Geometry check sheet. Reference: the model listing, model coordinates, mm. Face numbers are marked on the shaded views. Round coordinates to 2 decimals unless told otherwise and drop trailing zeros. Order: outer loops, then holes, each group sorted by start corner. A loop starts at its lowest first (then second) coordinate and runs counter-clockwise, first axis right, second up. Notation, with made-up numbers: (11.25, 46) - (43.25, 46) arc R8 ccw to (43.25, 52) - close; hole circle Ø10 at (40, 48). An arc over 180 degrees is marked (long way). Use a Markdown table: item, result. Add a question column.
(1) Section check D-D on x = 28.5. Record the boundary of the cut face in (y, z).
(2) Section check B-B on y = -22. Record the boundary of the cut face in (x, z), then the cut area to 3 significant figures.
(3) Gauge pin test, flat ends, axial feed: P1, Ø2, axis at y = 51.5, z = 2.5, coming from the -X side; P2, Ø1.5, axis at x = -49.5, z = 5, coming from the +Y side. Record the tip position at first contact, or that the pin passes through.
(4) Section check A-A on x = 0. Record the boundary of the cut face in (y, z).
(5) Mould release check, pull along X, two halves, no side actions. Record for the marked faces 1 and 2: released by +X, released by -X, zero draft, split by the parting line, or undercut.
(6) Thickness scan on line 1 along Z through (x, y) = (-29, 20); line 2 along Y through (x, z) = (7, 4.55); line 3 along Y through (x, z) = (15, 4.35). Record the ranges inside material, lowest first. Write a range as [from, to].
(7) Section check C-C on z = 1.65. Record the boundary of the cut face in (x, y).
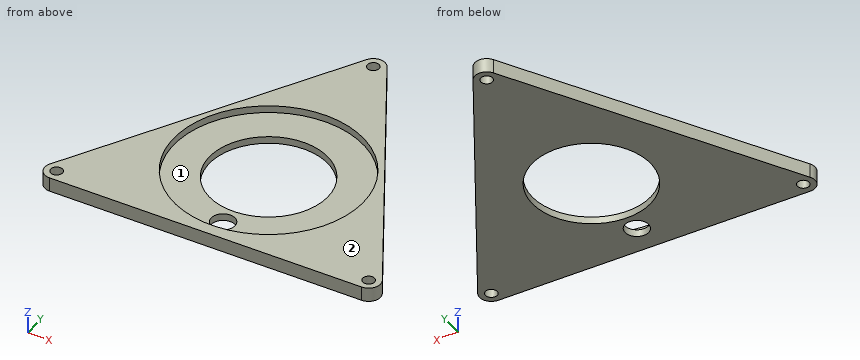
```python
from build123d import *

# Parameters (mm, degrees)
F0_R     = 2.5
F1_DEPTH = 6
F2_R     = 40
F3_DEPTH = 3
F4_R     = 25
F5_DEPTH = 25
F6_R     = 5
F7_DEPTH = 25


with BuildPart() as f1:
    # F0 (on Top) → F1 (new body)
    with BuildSketch(Plane.XY):
        with BuildLine():
            ThreePointArc((4.330127, 72.403811), (0, 74.903811), (-4.330127, 72.403811))
            Line((-4.330127, 72.403811), (-70.669873, -42.5))
            ThreePointArc((-70.669873, -42.5), (-70.669873, -47.5), (-66.339746, -50))
            Line((-66.339746, -50), (66.339746, -50))
            ThreePointArc((66.339746, -50), (70.669873, -47.5), (70.669873, -42.5))
            Line((70.669873, -42.5), (4.330127, 72.403811))
        make_face()
        with Locations((-66.339746, -45)):
            Circle(F0_R, mode=Mode.SUBTRACT)
        with Locations((66.339746, -45)):
            Circle(F0_R, mode=Mode.SUBTRACT)
        with Locations((0, 69.903811)):
            Circle(F0_R, mode=Mode.SUBTRACT)
    extrude(amount=F1_DEPTH)

    # F2 (on face) → F3 (cut)
    with BuildSketch(Plane.XY.offset(6)):
        with Locations((0, -5)):
            Circle(F2_R)
    extrude(amount=-F3_DEPTH, mode=Mode.SUBTRACT)

    # F4 (on face) → F5 (cut)
    with BuildSketch(Plane.XY.offset(3)):
        with Locations((0, -5)):
            Circle(F4_R)
    extrude(amount=-F5_DEPTH, mode=Mode.SUBTRACT)

    # F6 (on face) → F7 (cut)
    with BuildSketch(Plane.XY.offset(3)):
        with Locations((0, -37.5)):
            Circle(F6_R)
    extrude(amount=-F7_DEPTH, mode=Mode.SUBTRACT)


solid = f1.part
```
Check sheet entries:
| question | item | result |
|---|---|---|
| 1 | outline | (-50, 0) - (30.54, 0) - (30.54, 6) - (23.07, 6) - (23.07, 3) - (-33.07, 3) - (-33.07, 6) - (-50, 6) - close |
| 2 | outline | (-58.83, 0) - (-18.33, 0) - (-18.33, 3) - (-36.21, 3) - (-36.21, 6) - (-58.83, 6) - close; (18.33, 0) - (58.83, 0) - (58.83, 6) - (36.21, 6) - (36.21, 3) - (18.33, 3) - close |
| 2 | area | 379 mm2 |
| 3 | P1 | stops at x = -16.98 |
| 3 | P2 | stops at y = -4.53 |
| 4 | outline | (-50, 0) - (-42.5, 0) - (-42.5, 3) - (-45, 3) - (-45, 6) - (-50, 6) - close; (-32.5, 0) - (-30, 0) - (-30, 3) - (-32.5, 3) - close; (20, 0) - (67.4, 0) - (67.4, 6) - (35, 6) - (35, 3) - (20, 3) - close; (72.4, 0) - (74.9, 0) - (74.9, 6) - (72.4, 6) - close |
| 5 | face 1 | undercut |
| 5 | face 2 | zero draft |
| 6 | line 1 | z = [0, 3] |
| 6 | line 2 | y = [-50, -44.38], [34.38, 67.78] |
| 6 | line 3 | y = [-50, -42.08], [32.08, 53.92] |
| 7 | outline | (-70.67, -42.5) arc R5 ccw to (-66.34, -50) - (66.34, -50) arc R5 ccw to (70.67, -42.5) - (4.33, 72.4) arc R5 ccw to (-4.33, 72.4) - close; hole circle Ø5 at (-66.34, -45); hole circle Ø50 at (0, -5); hole circle Ø10 at (0, -37.5); hole circle Ø5 at (0, 69.9); hole circle Ø5 at (66.34, -45) |
